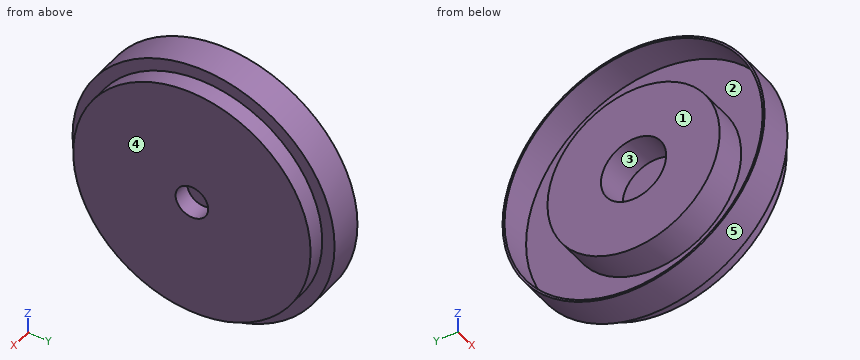
```python
from build123d import *

# Parameters (mm, degrees)
F1_W = 0.3
F1_H = 2.5


with BuildPart() as f3:
    # F0 (on Top) → F3 (revolve)
    with BuildSketch(Plane.XY):
        Polygon((0, 13.201755), (0, 5), (5, 5), (5, 2.5), (8, 2.5), (8, 18.201755), (5, 18.201755), (5, 13.201755), align=None)
    revolve(axis=Axis((9.429826, 0, 0), (1, 0, 0)))

    # F1 (on Top) → F4 (revolve)
    with BuildSketch(Plane.XY):
        with Locations((5.15, 1.25)):
            Rectangle(F1_W, F1_H)
        Polygon((5, 19.791724), (5, 18.201755), (5.3, 18.201755), (5.3, 20.091724), (0, 20.091724), (0, 19.791724), align=None)
    revolve(axis=Axis((9.429826, 0, 0), (1, 0, 0)))


solid = f3.part
```
Check sheet for the modelled part. Datum: model origin and axes. Units: mm. Face numbers are marked on the shaded views. A direction names the side the tool comes from. Give positions to 0.01 mm unless a question says otherwise; leave off trailing zeros. Loops run counter-clockwise (first coordinate to the right, second up) from the corner with the lowest first, then second, coordinate; pieces in that order, holes last. Notation, with made-up numbers: M 1,40 L 54,40 A36 cw 54,77 Z; hole C 47.5,61.5 d4. An arc over 180 degrees is marked long. Answer as CSV lines item,"result".
Item 1: Set-up check for the marked faces 1 and 2: record each of +Z, -Z, +X, -X, +Y, -Y from which the full face is reachable in a straight line by a thin tool's end or side.
Reply:
face 1,"+Z, -Z, -X, +Y, -Y"
face 2,"-X"
Item 2: Sectioned sample at D-D, the plane x = 7.25. Enter the section's corners in (y, z), then the cut area to 3 significant figures.
Reply:
outline,"C 0,0 d36.4; hole C 0,0 d5"
area,"1,020 mm^2"
Item 3: Sectioned sample at B-B, the plane x = 3.75. Enter the section's corners in (y, z).
Reply:
outline,"C 0,0 d40.18; C 0,0 d26.4; hole C 0,0 d39.58; hole C 0,0 d10"
Item 4: Sectioned sample at A-A, the plane z = 0. Enter the section's corners in (x, y).
Reply:
outline,"M 0,-20.09 L 5.3,-20.09 L 5.3,-18.2 L 8,-18.2 L 8,-2.5 L 5.3,-2.5 L 5.3,2.5 L 8,2.5 L 8,18.2 L 5.3,18.2 L 5.3,20.09 L 0,20.09 L 0,19.79 L 5,19.79 L 5,13.2 L 0,13.2 L 0,5 L 5,5 L 5,-5 L 0,-5 L 0,-13.2 L 5,-13.2 L 5,-19.79 L 0,-19.79 Z"
Item 5: Depth check by flat-ended pin: pin 1 Ø1 at (y, z) = (-11.5, 15) entering from +X; pin 2 Ø1 at (x, z) = (1, 14) entering from -Y; pin 3 Ø3 at (x, y) = (4, 15) entering from -Z. Enter the tip coordinate at first touch or a pass-through.
Reply:
pin 1,"x = 5.3"
pin 2,"y = -14.88"
pin 3,"z = -14.88"
Item 6: Draft check along Y on the marked faces 3, 4 and 5. Enter one of: pulls with the +Y half, pulls with the -Y half, needs draft (parallel to the pull), parting line crosses it, or undercut.
Reply:
face 3,"undercut"
face 4,"needs draft"
face 5,"parting line crosses it"
Item 7: Scan lines: L1, parallel to Z at x = 1.25, y = 0; L2, parallel to Z at x = 3.25, y = -1.5; L3, parallel to Z at x = 6.45, y = 0. Record each from-to range of solid material in increasing order.
Reply:
L1,"-20.09 to -19.79, -13.2 to -5, 5 to 13.2, 19.79 to 20.09"
L2,"-20.04 to -19.73, -13.12 to -4.77, 4.77 to 13.12, 19.73 to 20.04"
L3,"-18.2 to -2.5, 2.5 to 18.2"
